Work out the finished part from the listing and answer in its coordinate system (mm). Give positions to 0.01 mm unless a question says otherwise; leave off trailing zeros. Order: outer loops, then holes, each group sorted by start corner. A loop starts at its lowest first (then second) coordinate and runs counter-clockwise, first axis right, second up. Notation, with made-up numbers: (-24.75, -6.75) - (-3.75, -6.75) arc R21 ccw to (-3.75, 12.25) - close; hole circle Ø9 at (-16, 71). An arc over 180 degrees is marked (long way). Put each result on its own line as item: value.
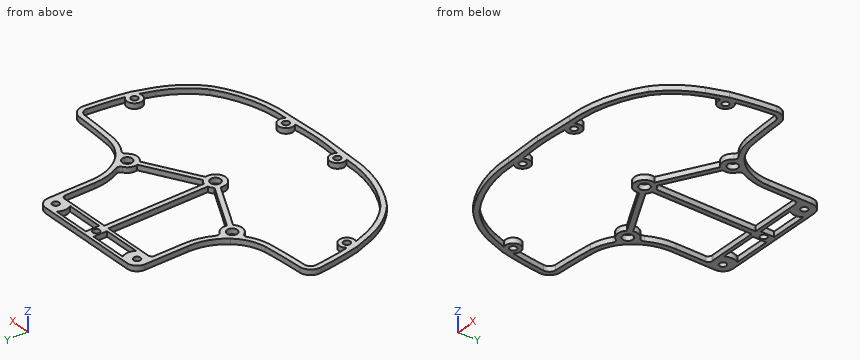
```python
from build123d import *

# Parameters (mm, degrees)
SKETCH4_R           = 1
SKETCH4_R_2         = 1.5
SKETCH4_R_3         = 1.500000001
BOSS_EXTRUDE2_DEPTH = 1.5875


with BuildPart() as part:
    # Sketch4 → Boss-Extrude2 (new body)
    with BuildSketch(Plane.XY):
        with BuildLine():
            ThreePointArc((-33.472754103, -25.121469845), (-23.054804413, -30.112701264), (-11.610361031, -31.68457355))
            Line((-11.610361031, -31.68457355), (0, -32.144613372))
            Line((0, -32.144613372), (11.610361031, -31.68457355))
            ThreePointArc((11.610361031, -31.68457355), (23.054804413, -30.112701264), (33.472754103, -25.121469845))
            ThreePointArc((33.472754103, -25.121469845), (38.084735692, -20.128369992), (41.315395383, -14.148047401))
            Line((41.315395383, -14.148047401), (43.310324676, -8.545068137))
            ThreePointArc((43.310324676, -8.545068137), (44.448650445, -2.324461154), (45.212741618, 3.953110149))
            ThreePointArc((45.212741618, 3.953110149), (44.453814547, 6.519739723), (42.09374947, 7.782138432))
            ThreePointArc((42.09374947, 7.782138432), (35.962680022, 8.111048014), (29.846780413, 8.653234381))
            ThreePointArc((29.846780413, 8.653234381), (25.580679904, 10.088760175), (22.077124707, 12.914613823))
            ThreePointArc((22.077124707, 12.914613823), (19.390258386, 17.570844388), (18.500000009, 22.872464303))
            Line((18.500000009, 22.872464303), (18.500000009, 35.75))
            ThreePointArc((18.500000009, 35.75), (17.62132035, 37.87132035), (15.5, 38.750000009))
            Line((15.5, 38.750000009), (-15.5, 38.750000009))
            ThreePointArc((-15.5, 38.750000009), (-17.62132035, 37.87132035), (-18.500000009, 35.75))
            Line((-18.500000009, 35.75), (-18.500000009, 22.872464277))
            ThreePointArc((-18.500000009, 22.872464277), (-19.390258383, 17.570844381), (-22.07712469, 12.91461383))
            ThreePointArc((-22.07712469, 12.91461383), (-25.580679805, 10.088760216), (-29.846780215, 8.653234395))
            ThreePointArc((-29.846780215, 8.653234395), (-35.962679941, 8.111048017), (-42.093749505, 7.78213843))
            ThreePointArc((-42.093749505, 7.78213843), (-44.453814559, 6.519739711), (-45.212741618, 3.953110149))
            ThreePointArc((-45.212741618, 3.953110149), (-44.448650445, -2.324461154), (-43.310324676, -8.545068137))
            Line((-43.310324676, -8.545068137), (-41.315395383, -14.148047401))
            ThreePointArc((-41.315395383, -14.148047401), (-38.084735692, -20.128369992), (-33.472754103, -25.121469845))
        make_face()
        with Locations((-9.815163292, -28.866300371)):
            Circle(SKETCH4_R, mode=Mode.SUBTRACT)
        with Locations((-40.488991371, -7.557479081)):
            Circle(SKETCH4_R, mode=Mode.SUBTRACT)
        with BuildLine():
            Line((-39.916947455, -13.605513167), (-41.326325711, -9.6458687))
            ThreePointArc((-41.326325711, -9.6458687), (-38.316546684, -6.971830651), (-42.262559751, -6.172937569))
            ThreePointArc((-42.262559751, -6.172937569), (-43.119549374, -1.052504396), (-43.720300768, 4.104274139))
            ThreePointArc((-43.720300768, 4.104274139), (-43.306279922, 5.553180603), (-41.988991391, 6.284955247))
            ThreePointArc((-41.988991391, 6.284955247), (-35.815859297, 6.617706074), (-29.658025423, 7.164848598))
            ThreePointArc((-29.658025423, 7.164848598), (-26.630229039, 7.954390182), (-23.847155024, 9.384574043))
            ThreePointArc((-23.847155024, 9.384574043), (-23.125480938, 9.525676377), (-22.515405804, 9.115150267))
            ThreePointArc((-22.515405804, 9.115150267), (-20.254015304, 7.760773306), (-17.79651867, 8.714153732))
            Line((-17.79651867, 8.714153732), (-2.913646, 0.714609672))
            ThreePointArc((-2.913646, 0.714609672), (0, -3), (2.913646001, 0.714609672))
            Line((2.913646001, 0.714609672), (17.79651867, 8.714153732))
            ThreePointArc((17.79651867, 8.714153732), (20.254015126, 7.760773291), (22.515405609, 9.115149969))
            ThreePointArc((22.515405609, 9.115149969), (23.125480765, 9.52567634), (23.847155026, 9.384574041))
            ThreePointArc((23.847155026, 9.384574041), (26.630229041, 7.954390183), (29.658025423, 7.164848601))
            ThreePointArc((29.658025423, 7.164848601), (35.815859287, 6.617706075), (41.988991371, 6.284955244))
            ThreePointArc((41.988991371, 6.284955244), (43.306279914, 5.553180608), (43.720300768, 4.104274139))
            ThreePointArc((43.720300768, 4.104274139), (43.119549374, -1.052504396), (42.262559751, -6.172937569))
            ThreePointArc((42.262559751, -6.172937569), (38.316546684, -6.971830651), (41.326325712, -9.6458687))
            Line((41.326325712, -9.6458687), (39.916947456, -13.605513167))
            ThreePointArc((39.916947456, -13.605513167), (36.88563151, -19.226390572), (32.562542901, -23.926820768))
            ThreePointArc((32.562542901, -23.926820768), (22.58818115, -28.686629582), (11.638338487, -30.184834485))
            ThreePointArc((11.638338487, -30.184834485), (9.815163292, -26.616300371), (7.991988098, -30.184834485))
            ThreePointArc((7.991988098, -30.184834485), (4.00190894, -30.517536934), (0, -30.644609524))
            ThreePointArc((0, -30.644609524), (-4.00190894, -30.517536934), (-7.991988097, -30.184834485))
            ThreePointArc((-7.991988097, -30.184834485), (-9.815163292, -26.616300371), (-11.638338487, -30.184834485))
            ThreePointArc((-11.638338487, -30.184834485), (-22.58818115, -28.686629582), (-32.562542901, -23.926820768))
            ThreePointArc((-32.562542901, -23.926820768), (-36.88563151, -19.226390572), (-39.916947455, -13.605513167))
        make_face(mode=Mode.SUBTRACT)
        with Locations((9.815163292, -28.866300371)):
            Circle(SKETCH4_R, mode=Mode.SUBTRACT)
        Circle(SKETCH4_R_2, mode=Mode.SUBTRACT)
        with Locations((40.488991371, -7.557479081)):
            Circle(SKETCH4_R, mode=Mode.SUBTRACT)
        with Locations((-20.000000001, 10.750000001)):
            Circle(SKETCH4_R_3, mode=Mode.SUBTRACT)
        with BuildLine():
            ThreePointArc((-18.952977672, 14.865256843), (-17.471741936, 18.750329795), (-17.000000007, 22.881347914))
            Line((-17.000000007, 22.881347914), (-17.000000007, 31.885058019))
            ThreePointArc((-17.000000007, 31.885058019), (-16.616434483, 32.496276684), (-15.954980266, 32.784701868))
            ThreePointArc((-15.954980266, 32.784701868), (-15.728150861, 32.758688041), (-15.5, 32.749999991))
            Line((-15.5, 32.749999991), (-0.750000001, 32.749999991))
            Line((-0.750000001, 32.749999991), (-0.750000001, 2.90473751))
            ThreePointArc((-0.750000001, 2.90473751), (-1.539319977, 2.574974565), (-2.20348133, 2.035846268))
            Line((-2.20348133, 2.035846268), (-17.086354, 10.035390328))
            ThreePointArc((-17.086354, 10.035390328), (-17.239112062, 11.923668519), (-18.492829269, 13.343922973))
            ThreePointArc((-18.492829269, 13.343922973), (-18.498254435, 13.347040523), (-18.503662642, 13.3501874))
            ThreePointArc((-18.503662642, 13.3501874), (-19.027733875, 14.018926796), (-18.952977672, 14.865256843))
        make_face(mode=Mode.SUBTRACT)
        with Locations((-15.5, 35.75)):
            Circle(SKETCH4_R, mode=Mode.SUBTRACT)
        with BuildLine():
            Line((-12.592865853, 37.75), (-1.5, 37.75))
            Line((-1.5, 37.75), (-1.5, 33.75))
            Line((-1.5, 33.75), (-12.612506492, 33.721747011))
            ThreePointArc((-12.612506492, 33.721747011), (-11.971383706, 35.732795451), (-12.592865853, 37.75))
        make_face(mode=Mode.SUBTRACT)
        with Locations((20, 10.75)):
            Circle(SKETCH4_R_2, mode=Mode.SUBTRACT)
        with BuildLine():
            Line((17.000000002, 31.88505801), (17.000000002, 22.881347906))
            ThreePointArc((17.000000002, 22.881347906), (17.471741935, 18.750329789), (18.952977675, 14.865256841))
            ThreePointArc((18.952977675, 14.865256841), (19.027733877, 14.018926793), (18.503662642, 13.350187397))
            ThreePointArc((18.503662642, 13.350187397), (18.498254436, 13.347040521), (18.492829272, 13.343922972))
            ThreePointArc((18.492829271, 13.343922974), (17.239112062, 11.923668519), (17.086354, 10.035390328))
            Line((17.086354, 10.035390328), (2.20348133, 2.035846268))
            ThreePointArc((2.20348133, 2.035846268), (1.539319976, 2.574974565), (0.749999999, 2.90473751))
            Line((0.749999999, 2.90473751), (0.749999999, 32.749999991))
            Line((0.749999999, 32.749999991), (15.5, 32.749999991))
            ThreePointArc((15.5, 32.749999991), (15.728150862, 32.758688041), (15.954980267, 32.784701869))
            ThreePointArc((15.954980267, 32.784701869), (16.616434482, 32.496276679), (17.000000002, 31.88505801))
        make_face(mode=Mode.SUBTRACT)
        with Locations((0, 35.75)):
            Circle(SKETCH4_R, mode=Mode.SUBTRACT)
        with BuildLine():
            Line((1.5, 33.75), (1.5, 37.75))
            Line((1.5, 37.75), (12.592865854, 37.75))
            ThreePointArc((12.592865854, 37.75), (11.971383706, 35.732795451), (12.612506492, 33.721747011))
            Line((12.612506492, 33.721747011), (1.5, 33.75))
        make_face(mode=Mode.SUBTRACT)
        with Locations((15.5, 35.75)):
            Circle(SKETCH4_R, mode=Mode.SUBTRACT)
    extrude(amount=BOSS_EXTRUDE2_DEPTH)


solid = part.part
```
(1) Given pin 1 (5 mm diameter, centred on x = 36, y = 5.5, fed in from -Z); pin 2 (0.5 mm diameter, centred on y = 31.5, z = 1, fed in from +X); pin 3 (1.8 mm diameter, centred on x = -15.5, y = 35.75, fed in from +Z); pin 4 (0.5 mm diameter, centred on x = 5, z = 0.5, fed in from -Y), each flat-ended and moving along its own axis, determine where each tip first touches the part or whether it passes through.
Geometry check:
pin 1: stops at z = 0
pin 2: stops at x = 18.5
pin 3: passes through
pin 4: stops at y = -31.96
(2) Section D-D, the plane x = 4 is taken. Write down the section's boundary in (y, z), then the cut area to 3 significant figures.
Geometry check:
outline: (-31.99, 0) - (-30.52, 0) - (-30.52, 1.59) - (-31.99, 1.59) - close; (1.3, 0) - (3, 0) - (3, 1.59) - (1.3, 1.59) - close; (32.75, 0) - (33.74, 0) - (33.74, 1.59) - (32.75, 1.59) - close; (37.75, 0) - (38.75, 0) - (38.75, 1.59) - (37.75, 1.59) - close
area: 8.20 mm²
(3) Straight lines are drawn through the part: line 1 (X direction, y = 21, z = 0.9); line 2 (X direction, y = -27, z = 0.3); line 3 (X direction, y = 23, z = 0.9). For each, find the intervals that lie inside material, in ascending order.
Geometry check:
line 1: x = -18.59 to -17.08, -0.75 to 0.75, 17.08 to 18.59
line 2: x = -30.44 to -27.1, -11.07 to -8.56, 8.56 to 11.07, 27.1 to 30.44
line 3: x = -18.5 to -17, -0.75 to 0.75, 17 to 18.5
(4) Section B-B, the plane x = -28.5 is taken. Write down the section's boundary in (y, z).
Geometry check:
outline: (-28, 0) - (-26.33, 0) - (-26.33, 1.59) - (-28, 1.59) - close; (7.38, 0) - (8.93, 0) - (8.93, 1.59) - (7.38, 1.59) - close
(5) Section C-C, the plane y = -15.5 is taken. Write down the section's boundary in (x, z).
Geometry check:
outline: (-40.75, 0) - (-39.09, 0) - (-39.09, 1.59) - (-40.75, 1.59) - close; (39.09, 0) - (40.75, 0) - (40.75, 1.59) - (39.09, 1.59) - close
(6) Section A-A, the plane y = 29 is taken. Write down the section's boundary in (x, z), then the cut area to 3 significant figures.
Geometry check:
outline: (-18.5, 0) - (-17, 0) - (-17, 1.59) - (-18.5, 1.59) - close; (-0.75, 0) - (0.75, 0) - (0.75, 1.59) - (-0.75, 1.59) - close; (17, 0) - (18.5, 0) - (18.5, 1.59) - (17, 1.59) - close
area: 7.14 mm²
